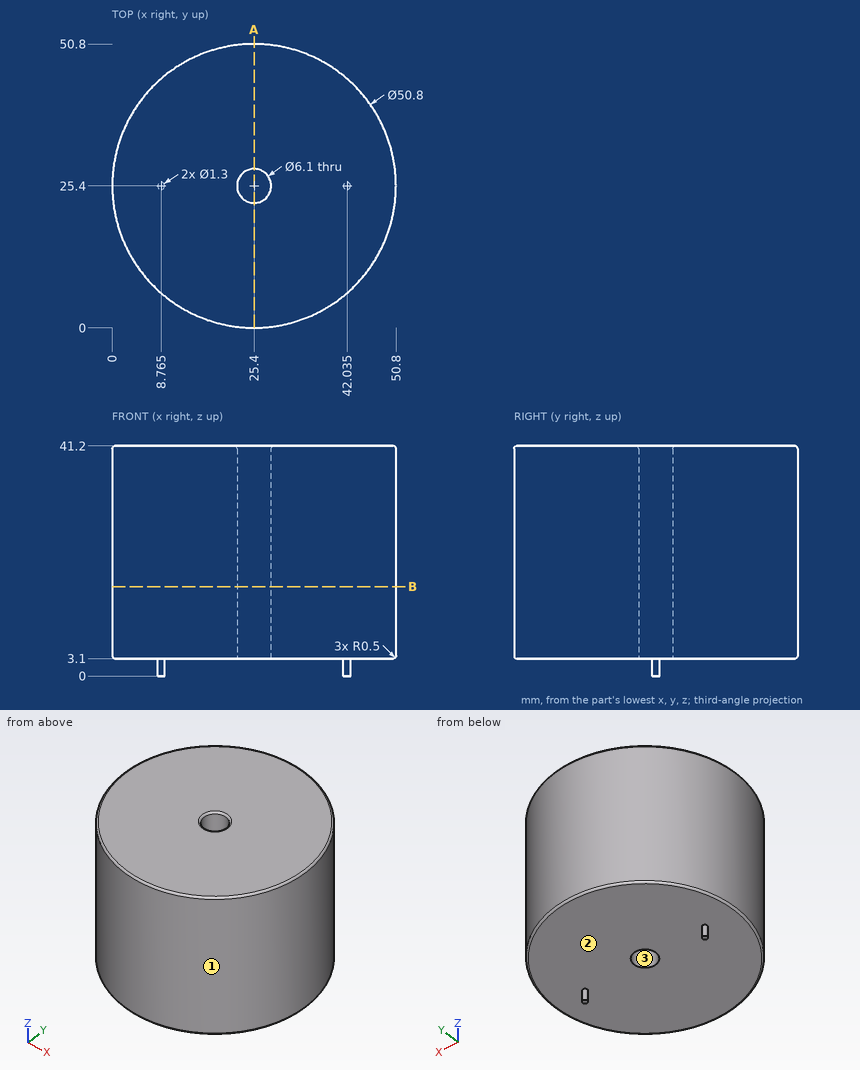
Can you work these out from the drawing? Everything is in mm from the part's minimum corner. Round coordinates to 2 decimals unless told otherwise and drop trailing zeros. Loops run counter-clockwise (first coordinate to the right, second up) from the corner with the lowest first, then second, coordinate; pieces in that order, holes last. Notation, with made-up numbers: (55, -11.5) - (113, -11.5) arc R17 cw to (113, 19.5) - close; hole circle Ø3 at (-34.5, 45). An arc over 180 degrees is marked (long way). Answer in a Markdown table with one row per item. Add a question column.
Q1. For pin 1 Ø2 at (y, z) = (22.5, 35) entering from -X; pin 2 Ø4 at (x, y) = (40, 28) entering from -Z; pin 3 Ø8 at (y, z) = (43.5, 11.5) entering from -X, each with a flat end and sliding along its axis, tell me the tip position at first contact or that it passes through.
Q2. We'd pull the mould along Y, two halves only. Please class the marked faces 1, 2 and 3: pulls with the +Y half, pulls with the -Y half, needs draft (parallel to the pull), parting line crosses it, or undercut.
Q3. I need wall thicknesses on L1, parallel to Y at x = 25.4, z = 24; L2, parallel to Z at x = 4, y = 28; L3, parallel to Y at x = 23, z = 29. Which ranges of each line are inside material? Lowest first, please.
Q4. I want a section at A-A on x = 25.4. List the corners of the cut face in (y, z) for me.
Q5. I want a section at B-B on z = 16. List the corners of the cut face in (x, y) for me.
A:
| question | item | result |
|---|---|---|
| 1 | pin 1 | x = 0.07 |
| 1 | pin 2 | z = 3.1 |
| 1 | pin 3 | x = 4.27 |
| 2 | face 1 | parting line crosses it |
| 2 | face 2 | needs draft |
| 2 | face 3 | undercut |
| 3 | L1 | 0 to 22.35, 28.45 to 50.8 |
| 3 | L2 | 3.1 to 41.2 |
| 3 | L3 | 0.11 to 23.52, 27.28 to 50.69 |
| 4 | outline | (0, 3.6) arc R0.5 ccw to (0.5, 3.1) - (22.35, 3.1) - (22.35, 40.7) arc R0.5 ccw to (21.85, 41.2) - (0.5, 41.2) arc R0.5 ccw to (0, 40.7) - close; (28.45, 3.1) - (50.3, 3.1) arc R0.5 ccw to (50.8, 3.6) - (50.8, 40.7) arc R0.5 ccw to (50.3, 41.2) - (28.95, 41.2) arc R0.5 ccw to (28.45, 40.7) - close |
| 5 | outline | circle Ø50.8 at (25.4, 25.4); hole circle Ø6.1 at (25.4, 25.4) |
